Could you check a few things on this drawing? It's one solid part, dimensions in mm from its lowest x, y, z. A direction names the side the tool comes from. Give positions to 0.01 mm unless a question says otherwise; leave off trailing zeros. Loops run counter-clockwise (first coordinate to the right, second up) from the corner with the lowest first, then second, coordinate; pieces in that order, holes last.
1. Imagine slicing it at D-D (z = 7.5). List the corners of the cut face in (x, y) for me, plus the area to 3 significant figures.
2. For P1, Ø2, axis at x = 14.5, z = 14, coming from the +Y side (1 decimal); P2, Ø2, axis at y = 12.5, z = 4.5, coming from the +X side; P3, Ø9, axis at x = 67.5, y = 7.5, coming from the +Z side, each with a flat end and sliding along its axis, tell me the tip position at first contact or that it passes through.
3. Imagine slicing it at A-A (z = 18). List the corners of the cut face in (x, y) for me, plus the area to 3 significant figures.
4. I need wall thicknesses on line 1 along Y through (x, z) = (67.5, 1.55); line 2 along X through (y, z) = (8.75, 2.75); line 3 along Z through (x, y) = (12.5, 11.25). Which ranges of each line are inside material? Lowest first, please.
5. Imagine slicing it at C-C (y = 3). List the corners of the cut face in (x, z) for me.
6. Imagine slicing it at B-B (x = 37.5). List the corners of the cut face in (y, z) for me.
7. Thinking about a two-plate mould opening in Y: for the marked faces 1, 2, 3 and 4, which applies, +Y half, -Y half, draft (parallel to the pull), parting line (faces both ways), or undercut?
8. For the marked faces 5, 6 and 7, which set-ups out of +Z, -Z, +X, -X, +Y, -Y let a thin tool reach every point of the face, with its end or its side?
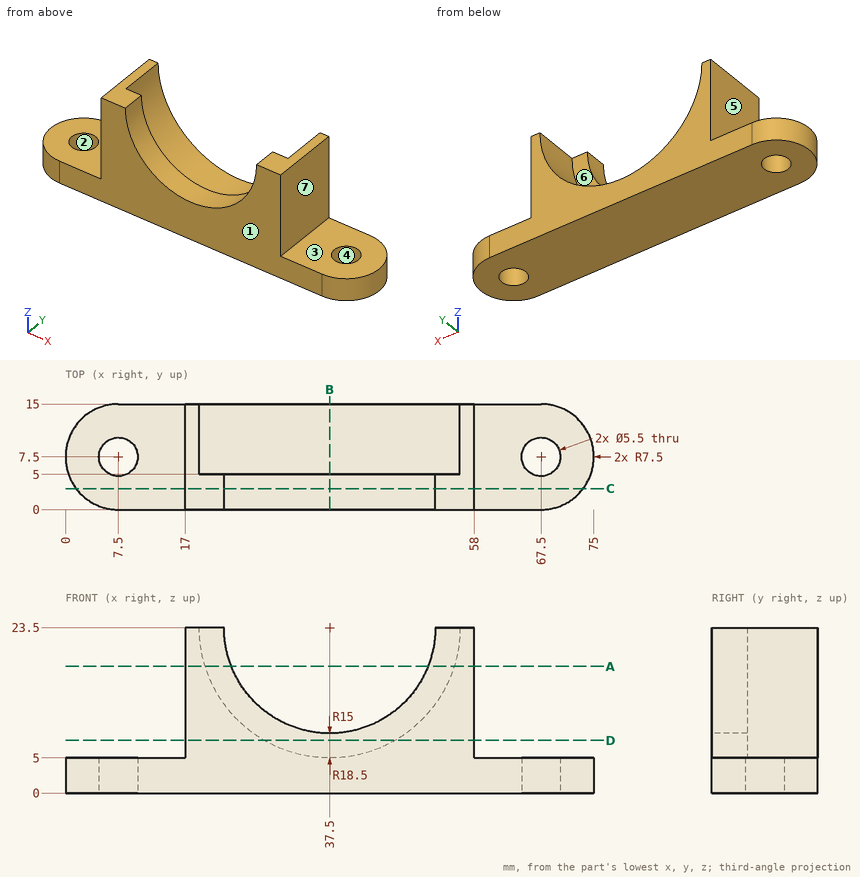
Derived:
1. outline: (17, 0) - (58, 0) - (58, 15) - (46.79, 15) - (46.79, 5) - (28.21, 5) - (28.21, 15) - (17, 15) - close
1. area: 429 mm2
2. P1: passes through
2. P2: stops at x = 73.84
2. P3: stops at z = 5
3. outline: (17, 0) - (23.54, 0) - (23.54, 5) - (19.84, 5) - (19.84, 15) - (17, 15) - close; (51.46, 0) - (58, 0) - (58, 15) - (55.16, 15) - (55.16, 5) - (51.46, 5) - close
3. area: 122 mm2
4. line 1: y = 0 to 4.75, 10.25 to 15
4. line 2: x = 0.1 to 5.05, 9.95 to 65.05, 69.95 to 74.9
4. line 3: z = 0 to 5
5. outline: (1.5, 0) - (73.5, 0) - (73.5, 5) - (58, 5) - (58, 23.5) - (52.5, 23.5) arc R15 cw to (22.5, 23.5) - (17, 23.5) - (17, 5) - (1.5, 5) - close
6. outline: (0, 0) - (15, 0) - (15, 5) - (5, 5) - (5, 8.5) - (0, 8.5) - close
7. face 1: -Y half
7. face 2: undercut
7. face 3: draft
7. face 4: undercut
8. face 5: +Z, -X, +Y, -Y
8. face 6: +Z, +Y
8. face 7: +Z, +X, +Y, -Y
